from build123d import *

# Parameters (mm, degrees)
F0_W      = 150
F0_H      = 60
F1_DEPTH  = 2
F2_W      = 2
F2_H      = 60
F3_DEPTH  = 30
F4_W      = 148
F4_H      = 2
F5_DEPTH  = 30
F6_W      = 2
F6_H      = 58
F7_DEPTH  = 30
F8_W      = 146
F8_H      = 2
F9_DEPTH  = 30
F11_W     = 2
F11_H     = 28
F12_DEPTH = 30
F13_W     = 80
F13_H     = 2
F14_DEPTH = 30
F16_W     = 1
F16_H     = 10
F17_DEPTH = 30
F18_W     = 28
F18_H     = 1
F19_DEPTH = 30
F20_W     = 1
F20_H     = 10
F21_DEPTH = 30
F22_W     = 1.5
F22_H     = 16
F23_DEPTH = 30
F24_W     = 1.5
F24_H     = 16
F25_DEPTH = 30
F26_W     = 7
F26_H     = 22
F27_DEPTH = 3
F28_W     = 6
F28_H     = 22
F29_DEPTH = 2


with BuildPart() as f1:
    # F0 (on Top) → F1 (new body)
    with BuildSketch(Plane.XY):
        with Locations((17.442032, 12.783553)):
            Rectangle(F0_W, F0_H)
    extrude(amount=F1_DEPTH)

    # F2 (on face) → F3 (join)
    with BuildSketch(Plane.XY.offset(2)):
        with Locations((-56.557968, 12.783553)):
            Rectangle(F2_W, F2_H)
    extrude(amount=F3_DEPTH)

    # F4 (on face) → F5 (join)
    with BuildSketch(Plane.XY.offset(2)):
        with Locations((18.442032, 41.783553)):
            Rectangle(F4_W, F4_H)
    extrude(amount=F5_DEPTH)

    # F6 (on face) → F7 (join)
    with BuildSketch(Plane.XY.offset(2)):
        with Locations((91.442032, 11.783553)):
            Rectangle(F6_W, F6_H)
    extrude(amount=F7_DEPTH)

    # F8 (on face) → F9 (join)
    with BuildSketch(Plane.XY.offset(2)):
        with Locations((17.442032, -16.216447)):
            Rectangle(F8_W, F8_H)
    extrude(amount=F9_DEPTH)

    # F11 (on face) → F12 (join)
    with BuildSketch(Plane.XY.offset(2)):
        with Locations((11.442032, 26.783553)):
            Rectangle(F11_W, F11_H)
    extrude(amount=F12_DEPTH)

    # F13 (on face) → F14 (join)
    with BuildSketch(Plane.XY.offset(2)):
        with Locations((50.442032, 13.783553)):
            Rectangle(F13_W, F13_H)
    extrude(amount=F14_DEPTH)

    # F16 (on face) → F17 (join)
    with BuildSketch(Plane.XY.offset(2)):
        with Locations((37.942032, 19.783553)):
            Rectangle(F16_W, F16_H)
    extrude(amount=F17_DEPTH)

    # F18 (on face) → F19 (join)
    with BuildSketch(Plane.XY.offset(2)):
        with Locations((51.442032, 24.283553)):
            Rectangle(F18_W, F18_H)
    extrude(amount=F19_DEPTH)

    # F20 (on face) → F21 (join)
    with BuildSketch(Plane.XY.offset(2)):
        with Locations((64.942032, 19.783553)):
            Rectangle(F20_W, F20_H)
    extrude(amount=F21_DEPTH)

    # F22 (on face) → F23 (join)
    with BuildSketch(Plane.XY.offset(2)):
        with Locations((46.192032, 32.783553)):
            Rectangle(F22_W, F22_H)
    extrude(amount=F23_DEPTH)

    # F24 (on face) → F25 (join)
    with BuildSketch(Plane.XY.offset(2)):
        with Locations((56.692032, 32.783553)):
            Rectangle(F24_W, F24_H)
    extrude(amount=F25_DEPTH)

    # F26 (on face) → F27 (cut)
    with BuildSketch(Plane.XZ.offset(-12.783553)):
        with Locations((51.942032, 13)):
            Rectangle(F26_W, F26_H)
    extrude(amount=-F27_DEPTH, mode=Mode.SUBTRACT)

    # F28 (on face) → F29 (cut)
    with BuildSketch(Plane.XZ.offset(-23.783553)):
        with Locations((52.442032, 13)):
            Rectangle(F28_W, F28_H)
    extrude(amount=-F29_DEPTH, mode=Mode.SUBTRACT)


solid = f1.part
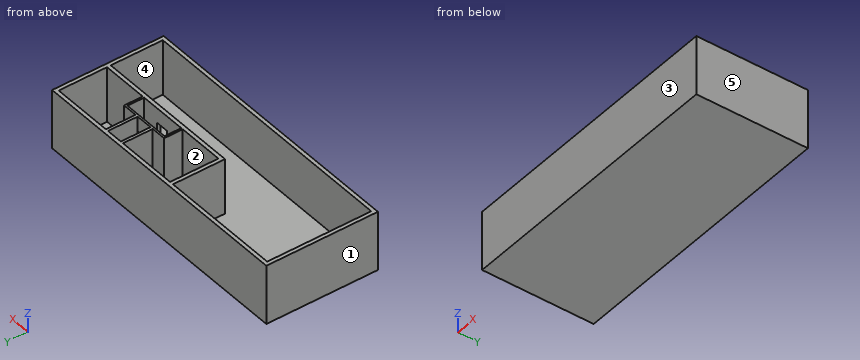
Build history of the part. All positions in model axes, mm. Face numbers are marked on the shaded views. A direction names the side the tool comes from. Round coordinates to 2 decimals unless told otherwise and drop trailing zeros. Loops run counter-clockwise (first coordinate to the right, second up) from the corner with the lowest first, then second, coordinate; pieces in that order, holes last. Notation, with made-up numbers: (63.5, 78.5) -> (98.5, 78.5) arc R29 ccw to (98.5, 103.5) -> close; hole circle Ø7 at (-27, 71.25). An arc over 180 degrees is marked (long way). Use CSV: the item, a comma, the result in double quotes. Start each with the question number.
Q1. Saw through at A-A on z = 29. Count the separate pieces of the cut face and the enclosed holes in it, and give its area (3 significant figures).
Q2. Saw through at B-B on x = 8. Give the cut face in (y, z), and give its area (3 significant figures).
Q3. Which spindle directions (+Z, -Z, +X, -X, +Y, -Y) get a long thin tool onto all of the face, cutting with end or side? Do the marked faces 1 and 2. Say none if no direction does.
Q4. Saw through at D-D on y = 20. Give the cut face in (x, z), and give its area (3 significant figures).
Q5. Flat gauge pin, fed straight in: pin 1 Ø8 at (x, y) = (22, 33.5) entering from -Z. Where does the tip first touch, or does it go through?
Q6. Drill centre lines: L1, parallel to X at y = 16, z = 21.5; L2, parallel to Y at x = 31.5, z = 3.5; L3, parallel to X at y = 26, z = 3. Where is each one in solid material? Low to high.
Q7. Saw through at C-C on y = 36.5. Give the cut face in (x, z), and give its area (3 significant figures).
Q8. Mould opens along Y. For the marked faces 3, 4 and 5 say: +Y half, -Y half, draft (parallel to the pull), parting line (faces both ways), or undercut.
Solutions:
1,separate pieces,"1"
1,enclosed holes,"5"
1,area,"1,130 mm^2"
2,outline,"(-17.22, 0) -> (42.78, 0) -> (42.78, 32) -> (40.78, 32) -> (40.78, 2) -> (-15.22, 2) -> (-15.22, 32) -> (-17.22, 32) -> close"
2,area,"240 mm^2"
3,face 1,"+Z, -Z, -X, +Y, -Y"
3,face 2,"+Z"
4,outline,"(-57.56, 0) -> (92.44, 0) -> (92.44, 32) -> (90.44, 32) -> (90.44, 2) -> (65.44, 2) -> (65.44, 32) -> (64.44, 32) -> (64.44, 2) -> (38.44, 2) -> (38.44, 32) -> (37.44, 32) -> (37.44, 2) -> (12.44, 2) -> (12.44, 32) -> (10.44, 32) -> (10.44, 2) -> (-55.56, 2) -> (-55.56, 32) -> (-57.56, 32) -> close"
4,area,"540 mm^2"
5,pin 1,"stops at z = 0"
6,L1,"x = -57.56 to -55.56, 10.44 to 12.44, 37.44 to 38.44, 64.44 to 65.44, 90.44 to 92.44"
6,L2,"y = -17.22 to -15.22, 12.78 to 14.78, 40.78 to 42.78"
6,L3,"x = -57.56 to -55.56, 10.44 to 12.44, 45.44 to 46.94, 55.94 to 57.44, 90.44 to 92.44"
7,outline,"(-57.56, 0) -> (92.44, 0) -> (92.44, 32) -> (90.44, 32) -> (90.44, 2) -> (57.44, 2) -> (57.44, 32) -> (55.94, 32) -> (55.94, 2) -> (46.94, 2) -> (46.94, 32) -> (45.44, 32) -> (45.44, 2) -> (12.44, 2) -> (12.44, 32) -> (10.44, 32) -> (10.44, 2) -> (-55.56, 2) -> (-55.56, 32) -> (-57.56, 32) -> close"
7,area,"570 mm^2"
8,face 3,"-Y half"
8,face 4,"undercut"
8,face 5,"draft"
